Input: part model. Units: mm. Frame: model coordinates. Coordinates: 2 decimals unless noted, no trailing zeros. Write each loop counter-clockwise with the first axis right and the second up, starting at its lowest first coordinate (ties: lowest second). Pieces come first, ordered by that corner, then holes. Notation, with made-up numbers: (-2.5, 5.5) - (21.5, 5.5) arc R12 ccw to (21.5, 14.5) - close; hole circle Ø4 at (67, 88.5). An arc over 180 degrees is marked (long way). Use CSV: the item, a comma, the result in double quotes.
```python
from build123d import *

# Parameters (mm, degrees)
BASE_DEPTH         = 5.334
CUT_EXTRUDE1_REACH = 7.334
SKETCH3_W          = 25.4
SKETCH3_H          = 10.668


with BuildPart() as part:
    # Sketch1 → Base (new body)
    with BuildSketch(Plane(origin=(0, 0, 0), x_dir=(1, 0, 0), z_dir=(0, 1, 0))):
        Polygon((0, 0), (380.417035208, -21.068443786), (380.417035208, -103.983742074), (0, -170.235385513), align=None)
    extrude(amount=BASE_DEPTH)

    # Sketch3 → Cut-Extrude1 (cut, up to next)
    with BuildSketch(Plane.XZ, mode=Mode.PRIVATE) as cut_extrude1_sk1:
        with Locations((278.817035208, 59.945526857)):
            Rectangle(SKETCH3_W, SKETCH3_H)
    cut_extrude1_tool1 = extrude(cut_extrude1_sk1.sketch, amount=-CUT_EXTRUDE1_REACH, mode=Mode.PRIVATE) & part.part
    add(cut_extrude1_tool1.solids().sort_by_distance((278.817035, 0, 59.945527))[0], mode=Mode.SUBTRACT)
    # Sketch3 → Cut-Extrude1 (cut, up to next)
    with BuildSketch(Plane.XZ, mode=Mode.PRIVATE) as cut_extrude1_sk2:
        with Locations((88.9, 59.945526857)):
            Rectangle(SKETCH3_W, SKETCH3_H)
    cut_extrude1_tool2 = extrude(cut_extrude1_sk2.sketch, amount=-CUT_EXTRUDE1_REACH, mode=Mode.PRIVATE) & part.part
    add(cut_extrude1_tool2.solids().sort_by_distance((88.9, 0, 59.945527))[0], mode=Mode.SUBTRACT)


solid = part.part
```
(1) Cut plane C-C on z = 139.5. Return loops of the section in (x, y).
Check values:
outline,"(0, 0) - (176.48, 0) - (176.48, 5.33) - (0, 5.33) - close"
(2) Cut plane D-D on x = 41.5. Return loops of the section in (y, z), and give its area (3 significant figures).
Check values:
outline,"(0, 2.3) - (5.33, 2.3) - (5.33, 163.01) - (0, 163.01) - close"
area,"857 mm^2"
(3) Cut plane A-A on x = 281. Return loops of the section in (y, z).
Check values:
outline,"(0, 15.56) - (5.33, 15.56) - (5.33, 54.61) - (0, 54.61) - close; (0, 65.28) - (5.33, 65.28) - (5.33, 121.3) - (0, 121.3) - close"
(4) Cut plane B-B on y = 3.6. Return loops of the section in (x, z), and give its area (3 significant figures).
Check values:
outline,"(0, 0) - (380.42, 21.07) - (380.42, 103.98) - (0, 170.24) - close; hole (76.2, 54.61) - (101.6, 54.61) - (101.6, 65.28) - (76.2, 65.28) - close; hole (266.12, 54.61) - (291.52, 54.61) - (291.52, 65.28) - (266.12, 65.28) - close"
area,"47,600 mm^2"
(5) Pin query (flat end, axial travel): pin 1 Ø2 at (x, y) = (196, 3) entering from +Z; pin 2 Ø3 at (y, z) = (2.5, 43) entering from -X; pin 3 Ø2.5 at (x, y) = (276.5, 2) entering from -Z; pin 4 Ø3 at (x, y) = (335.5, 1) entering from -Z. Return the tip coordinate at first contact, or that it passes through.
Check values:
pin 1,"z = 136.28"
pin 2,"x = 0"
pin 3,"z = 15.24"
pin 4,"z = 18.5"
(6) Ray query, probe 1 along X at (y, z) = (4.85, 65); probe 2 along Z at (x, y) = (273, 3.4); probe 3 along Z at (x, y) = (267, 1.4). Return the intervals inside material, ascending. Write a range as from..to.
Check values:
probe 1,"0..76.2, 101.6..266.12, 291.52..380.42"
probe 2,"15.12..54.61, 65.28..122.69"
probe 3,"14.79..54.61, 65.28..123.74"
